from build123d import *

# Parameters (mm, degrees)
BOSS_EXTRUDE1_DEPTH = 1.524


with BuildPart() as part:
    # Sketch1 → Boss-Extrude1 (new body)
    with BuildSketch(Plane.XY):
        with BuildLine():
            Line((0.758413423, -14.514612412), (0.756426596, -5.229573284))
            Line((0.756426596, -5.229573284), (-0.767567777, -5.228579871))
            Line((-0.767567777, -5.228579871), (-0.767567777, -14.513618998))
            ThreePointArc((-0.767567777, -14.513618998), (-1.539192536, -14.521879258), (-2.263766939, -14.78733158))
            ThreePointArc((-2.263766939, -14.78733158), (-3.206305559, -13.566940945), (-3.825331329, -12.1546593))
            ThreePointArc((-3.825331329, -12.1546593), (-3.623089301, -15.369727095), (-2.663937168, -18.445046583))
            ThreePointArc((-2.663937168, -18.445046583), (-1.772934243, -19.968018634), (-1.903339021, -21.727656288))
            ThreePointArc((-1.903339021, -21.727656288), (-3.266929983, -25.997412135), (-4.052166969, -30.410302139))
            ThreePointArc((-4.052166969, -30.410302139), (-5.395158951, -25.68457677), (-7.349213338, -21.177052042))
            ThreePointArc((-7.349213338, -21.177052042), (-7.559215071, -20.612929546), (-7.63057286, -20.015231476))
            Line((-7.63057286, -20.015231476), (-7.631892886, 4.626897175))
            ThreePointArc((-7.631892886, 4.626897175), (-7.092287621, 5.859442088), (-5.820556253, 6.298805414))
            ThreePointArc((-5.820556253, 6.298805414), (-4.085125664, 6.930306858), (-3.428174811, 8.656264268))
            Line((-3.428174811, 8.656264268), (-3.431470931, 20.183759219))
            ThreePointArc((-3.431470931, 20.183759219), (-3.418767766, 20.417805376), (-3.390090239, 20.650435067))
            ThreePointArc((-3.390090239, 20.650435067), (-6.519567928, 26.925166891), (-13.182414969, 29.109739933))
            ThreePointArc((-13.182414969, 29.109739933), (-14.180468361, 30.396049042), (-13.396765315, 31.823112892))
            ThreePointArc((-13.396765315, 31.823112892), (-8.064833076, 33.586641612), (-3.820754211, 29.9086898))
            ThreePointArc((-3.820754211, 29.9086898), (-3.115822585, 27.98554328), (-2.136235135, 26.186702108))
            ThreePointArc((-2.136235135, 26.186702108), (-0.000993472, 25.022326708), (2.134248191, 26.186702108))
            ThreePointArc((2.134248191, 26.186702108), (3.113835641, 27.98554328), (3.818767267, 29.9086898))
            ThreePointArc((3.818767267, 29.9086898), (8.062846132, 33.586641612), (13.394778371, 31.823112892))
            ThreePointArc((13.394778371, 31.823112892), (14.178481417, 30.396049042), (13.180428025, 29.109739933))
            ThreePointArc((13.180428025, 29.109739933), (6.517580984, 26.925166891), (3.388103295, 20.650435067))
            ThreePointArc((3.388103295, 20.650435067), (3.412047002, 20.417632477), (3.420040198, 20.183738364))
            Line((3.420040198, 20.183738364), (3.421535659, 8.656441281))
            ThreePointArc((3.421535659, 8.656441281), (4.079205123, 6.93199833), (5.813550357, 6.300904656))
            ThreePointArc((5.813550357, 6.300904656), (7.087362904, 5.86275757), (7.628225836, 4.6290483))
            Line((7.628225836, 4.6290483), (7.631801236, -20.008478102))
            ThreePointArc((7.631801236, -20.008478102), (7.56045, -20.606653876), (7.350236218, -21.171202742))
            ThreePointArc((7.350236218, -21.171202742), (5.394278235, -25.681479256), (4.050180025, -30.410302139))
            ThreePointArc((4.050180025, -30.410302139), (3.265080471, -25.998057724), (1.901795058, -21.728896802))
            ThreePointArc((1.901795058, -21.728896802), (1.770271466, -19.970622492), (2.657373106, -18.446851614))
            ThreePointArc((2.657373106, -18.446851614), (3.616525238, -15.371532126), (3.818767267, -12.156464331))
            ThreePointArc((3.818767267, -12.156464331), (3.199964786, -13.568369499), (2.257818447, -14.788514159))
            ThreePointArc((2.257818447, -14.788514159), (1.531710448, -14.522401162), (0.758413423, -14.514612412))
        make_face()
    extrude(amount=BOSS_EXTRUDE1_DEPTH)


solid = part.part
Here's how the part is built. I have some questions about the finished solid (model axes, mm). A direction names the side the tool comes from. Round coordinates to 2 decimals unless told otherwise and drop trailing zeros. Loops run counter-clockwise (first coordinate to the right, second up) from the corner with the lowest first, then second, coordinate; pieces in that order, holes last. Notation, with made-up numbers: (57, -23.5) -> (106, -23.5) arc R19 cw to (106, -9.5) -> close; hole circle Ø3 at (54, -15). An arc over 180 degrees is marked (long way). Write each question's results on one line, items separated by ' | '.
(1) If we section it at B-B, the plane x = 9.5: List the corners of the cut face in (y, z) for me, then the cut area to 3 significant figures.
Worked answers:
outline: (28.64, 0) -> (33.69, 0) -> (33.69, 1.52) -> (28.64, 1.52) -> close | area: 7.69 mm2
(2) If we section it at C-C, the plane y = -8: List the corners of the cut face in (x, z) for me, then the cut area to 3 significant figures.
Worked answers:
outline: (-7.63, 0) -> (-0.77, 0) -> (-0.77, 1.52) -> (-7.63, 1.52) -> close; (0.76, 0) -> (7.63, 0) -> (7.63, 1.52) -> (0.76, 1.52) -> close | area: 20.9 mm2
(3) If I drill on L1, parallel to X at y = -10.5, z = 1.15; L2, parallel to X at y = 0, z = 0.9; L3, parallel to X at y = 26, z = 0.6, over which ranges is the centre line in solid material (lowest first)?
Worked answers:
L1: -7.63 to -0.77, 0.76 to 7.63 | L2: -7.63 to 7.63 | L3: -5.59 to -2, 2 to 5.59
(4) We'd pull the mould along Y, two halves only. Please class faces 4 (the face through (-7.106, 5.846, 0.751)), 5 (the face through (-6.444, 26.859, 0.751)), 6 (the face through (-5.37, -25.75, 0.75)), 7 (the face through (14.18, 30.42, 0.75)): released by +Y, released by -Y, zero draft, split by the parting line, or undercut.
Worked answers:
face 4: undercut | face 5: undercut | face 6: released by -Y | face 7: split by the parting line
(5) For faces 1 (the face through (-3.128, 28.012, 0.751)), 2 (the face through (3.28, -26.06, 0.75)), 3 (the face through (1.542, -14.524, 0.751)), which set-ups out of +Z, -Z, +X, -X, +Y, -Y let a thin tool reach every point of the face, with its end or its side?
Worked answers:
face 1: +Z, -Z, +Y | face 2: +Z, -Z, -Y | face 3: +Z, -Z
(6) For P1, Ø0.5, axis at y = 14.5, z = 1, coming from the +X side; P2, Ø0.5, axis at y = 16, z = 0.5, coming from the -X side; P3, Ø0.5, axis at y = -9.5, z = 0.5, coming from the -X side, each with a flat end and sliding along its axis, tell me the tip position at first contact or that it passes through.
Worked answers:
P1: x = 3.42 | P2: x = -3.43 | P3: x = -7.63
(7) If we section it at A-A, the plane y = -17.5: List the corners of the cut face in (x, z) for me, then the cut area to 3 significant figures.
Worked answers:
outline: (-7.63, 0) -> (-3.05, 0) -> (-3.05, 1.52) -> (-7.63, 1.52) -> close; (3.04, 0) -> (7.63, 0) -> (7.63, 1.52) -> (3.04, 1.52) -> close | area: 14.0 mm2
(8) If we section it at D-D, the plane y = 19.5: List the corners of the cut face in (x, z) for me, then the cut area to 3 significant figures.
Worked answers:
outline: (-3.43, 0) -> (3.42, 0) -> (3.42, 1.52) -> (-3.43, 1.52) -> close | area: 10.4 mm2
